Source: CAD feature listing. Evaluate the final solid. Frame: model axes, mm. Face numbers are marked on the shaded views. A direction names the side the tool comes from. Round coordinates to 2 decimals unless told otherwise and drop trailing zeros. Loops run counter-clockwise (first coordinate to the right, second up) from the corner with the lowest first, then second, coordinate; pieces in that order, holes last. Notation, with made-up numbers: M 76,-22 L 103,-22 A22 ccw 103,-8 Z; hole C 41,37 d6. An arc over 180 degrees is marked long. Write each question's results on one line, items separated by ' | '. Start each with the question number.
1. Set-up query: the marked faces 1 and 2. Return all of +Z, -Z, +X, -X, +Y, -Y with unobstructed straight access to the full face (end or side cutting, diameter ignored); none if empty.
2. Section A-A on y = 9. Give the number of separate pieces and of enclosed holes in the cut face, and give its area (3 significant figures).
3. Ray query, line 1 (Z direction, x = -50.5, y = 7.25) (3 decimals); line 2 (Y direction, x = -40.5, z = -7); line 3 (X direction, y = 8.75, z = -10.5) (3 decimals). Return the intervals inside material, ascending.
4. Contact query for flat-ended pins moving along their axis: pin 1 Ø1.6 at (x, y) = (-71, 9.5) entering from -Z (3 decimals); pin 2 Ø3.5 at (x, z) = (-78, -39) entering from +Y; pin 3 Ø3 at (y, z) = (8, -67.5) entering from +X (3 decimals). Output: stop coordinate, or through.
5. Section B-B on z = -12.5. Output: boundary loops of the cut face in (x, y) (3 decimals).
6. Section D-D on z = -36.5. Output: boundary loops of the cut face in (x, y) (3 decimals).
7. Draft query along X for the marked faces 3 and 4. Return one class per face: released by +X, released by -X, zero draft, split by the parting line, or undercut.
Autodesk Inventor part; units mm, degrees
ref_plane "YZ Plane" through (0, 0, 0) normal (1, 0, 0) x (0, 1, 0)
ref_plane "XZ Plane" through (0, 0, 0) normal (0, 1, 0) x (-1, 0, 0)
ref_plane "XY Plane" through (0, 0, 0) normal (0, 0, 1) x (1, 0, 0)
sketch "Boceto1" plane through (0, 0, 0) normal (0, 1, 0) x (-1, 0, 0)
  line L0 (0, 0) -> (80, 0)
  line L1 (80, 0) -> (80, -80)
  line L2 (80, -80) -> (0, -80)
  line L3 (0, -80) -> (0, 0)
  line L4 (10, -70) -> (70, -70)
  line L5 (70, -70) -> (70, -10)
  line L6 (70, -10) -> (10, -10)
  line L7 (10, -10) -> (10, -70)
  line L8 (0, -12.375) -> (80, -12.375)
  line L9 (0, -14.95) -> (80, -14.95)
  line L10 (0, -17.525) -> (80, -17.525)
  line L11 (80, -20.1) -> (0, -20.1)
  line L12 (0, -22.675) -> (80, -22.675)
  line L13 (0, -12.575) -> (80, -12.575)
  line L14 (0, -15.15) -> (80, -15.15)
  line L15 (0, -17.725) -> (80, -17.725)
  line L16 (80, -20.3) -> (0, -20.3)
  line L17 (0, -22.875) -> (80, -22.875)
  line L18 (0, -25.25) -> (80, -25.25)
  line L19 (0, -25.45) -> (80, -25.45)
  line L20 (10, -40) -> (80, -40)
  line L21 (0, -67.625) -> (80, -67.625)
  line L22 (0, -65.05) -> (80, -65.05)
  line L23 (0, -62.475) -> (80, -62.475)
  line L24 (80, -59.9) -> (0, -59.9)
  line L25 (0, -57.325) -> (80, -57.325)
  line L26 (0, -67.425) -> (80, -67.425)
  line L27 (0, -64.85) -> (80, -64.85)
  line L28 (0, -62.275) -> (80, -62.275)
  line L29 (80, -59.7) -> (0, -59.7)
  line L30 (0, -57.125) -> (80, -57.125)
  line L31 (0, -54.75) -> (80, -54.75)
  line L32 (0, -54.55) -> (80, -54.55)
  line L33 (72.625, -7.375) -> (7.375, -7.375)
  line L34 (7.375, -7.375) -> (7.375, -72.625)
  line L35 (7.375, -72.625) -> (72.625, -72.625)
  line L36 (72.625, -72.625) -> (72.625, -7.375)
  line L37 (7.375, 0) -> (0, 0)
  line L38 (7.375, -80) -> (0, -80)
  point P0 (10, -12.375)
  point P1 (70, -12.375)
  point P2 (10, -14.95)
  point P3 (70, -14.95)
  point P4 (10, -17.525)
  point P5 (70, -17.525)
  point P6 (70, -20.1)
  point P7 (10, -20.1)
  point P8 (10, -22.675)
  point P9 (70, -22.675)
  point P10 (10, -12.575)
  point P11 (70, -12.575)
  point P12 (10, -15.15)
  point P13 (70, -15.15)
  point P14 (10, -17.725)
  point P15 (70, -17.725)
  point P16 (70, -20.3)
  point P17 (10, -20.3)
  point P18 (10, -22.875)
  point P19 (70, -22.875)
  point P20 (10, -25.25)
  point P21 (70, -25.25)
  point P22 (10, -25.45)
  point P23 (70, -25.45)
  point P24 (10, -67.625)
  point P25 (70, -67.625)
  point P26 (10, -65.05)
  point P27 (70, -65.05)
  point P28 (10, -62.475)
  point P29 (70, -62.475)
  point P30 (70, -59.9)
  point P31 (10, -59.9)
  point P32 (10, -57.325)
  point P33 (70, -57.325)
  point P34 (10, -67.425)
  point P35 (70, -67.425)
  point P36 (10, -64.85)
  point P37 (70, -64.85)
  point P38 (10, -62.275)
  point P39 (70, -62.275)
  point P40 (70, -59.7)
  point P41 (10, -59.7)
  point P42 (10, -57.125)
  point P43 (70, -57.125)
  point P44 (10, -54.75)
  point P45 (70, -54.75)
  point P46 (10, -54.55)
  point P47 (70, -54.55)
  point P48 (72.625, -12.375)
  point P49 (7.375, -12.375)
  point P50 (72.625, -54.55)
  point P51 (72.625, -25.45)
  point P52 (70, -25.45)
  point P53 (70, -54.55)
  point P54 (7.375, -25.45)
  point P55 (7.375, -54.55)
  point P56 (10, -54.55)
  point P57 (10, -25.45)
  point P58 (10, -67.625)
  point P59 (7.375, -67.625)
  point P60 (72.625, -67.625)
  point P61 (70, -67.625)
  point P62 (7.375, -14.95)
  point P63 (72.625, -14.95)
  point P64 (72.625, -65.05)
  point P65 (70, -65.05)
  point P66 (10, -65.05)
  point P67 (7.375, -65.05)
  point P68 (70, -67.425)
  point P69 (10, -67.425)
  point P70 (10, -12.575)
  point P71 (70, -12.575)
  point P72 (72.625, -64.85)
  point P73 (7.375, -64.85)
  point P74 (7.375, -15.15)
  point P75 (70, -15.15)
  point P76 (7.375, -62.475)
  point P77 (10, -64.85)
  point P78 (10, -62.475)
  point P79 (72.625, -62.475)
  point P80 (70, -62.475)
  point P81 (70, -64.85)
  point P82 (7.375, -17.525)
  point P83 (10, -15.15)
  point P84 (72.625, -17.525)
  point P85 (72.625, -20.1)
  point P86 (7.375, -20.1)
  point P87 (72.625, -59.9)
  point P88 (70, -59.9)
  point P89 (70, -62.275)
  point P90 (10, -62.275)
  point P91 (10, -59.9)
  point P92 (7.375, -59.9)
  point P93 (10, -17.725)
  point P94 (70, -17.725)
  dimension "d0" = 80
  dimension "d1" = 80
  dimension "d2" = 60
  dimension "d3" = 60
  dimension "d4" = 10
  dimension "d5" = 10
  dimension "d6" = 2.375
  dimension "d7" = 0.2
  dimension "d8" = 2.375
  dimension "d9" = 0.2
  dimension "d10" = 0.2
  dimension "d11" = 0.2
  dimension "d12" = 0.2
  dimension "d13" = 2.375
  dimension "d14" = 2.375
  dimension "d15" = 2.375
  dimension "d16" = 2.375
  dimension "d17" = 0.2
  dimension "d35" = 5
extrude "Extrusión1" add sketch "Boceto1" along normal blind 5 contours L0 L1 L8 L36 L33 L34 L3 | L8 L34 L13 L3 | L13 L34 L9 L3 | L34 L33 L36 L8 L5 L6 L7 | L8 L7 L13 L34 | L1 L13 L36 L8 | L13 L7 L9 L34 | L8 L5 L13 L7 | L7 L6 L5 L8 | L1 L9 L36 L13 | L36 L13 L5 L8 | L14 L34 L10 L3 | L13 L5 L9 L7 | L36 L9 L5 L13 | L14 L7 L10 L34 | L1 L10 L36 L14 | L15 L34 L11 L3 | L14 L5 L10 L7 | L36 L10 L5 L14 | L15 L7 L11 L34 | L1 L11 L36 L15 | L16 L34 L12 L3 | L15 L5 L11 L7 | L36 L11 L5 L15 | L16 L7 L12 L34 | L1 L12 L36 L16 | L17 L34 L18 L3 | L16 L5 L12 L7 | L36 L12 L5 L16 | L17 L7 L18 L34 | L1 L18 L36 L17 | L19 L34 L32 L3 | L17 L5 L18 L7 | L36 L18 L5 L17 | L19 L7 L32 L34 | L1 L20 L36 L19 | L31 L34 L30 L3 | L19 L5 L20 L7 | L1 L32 L36 L20 | L36 L20 L5 L19 | L31 L7 L30 L34 | L7 L20 L5 L32 | L36 L32 L5 L20 | L25 L34 L29 L3 | L31 L5 L30 L7 | L1 L30 L36 L31 | L25 L7 L29 L34 | L31 L36 L30 L5 | L24 L34 L28 L3 | L25 L5 L29 L7 | L1 L29 L36 L25 | L24 L7 L28 L34 | L25 L36 L29 L5 | L23 L34 L27 L3 | L24 L5 L28 L7 | L1 L28 L36 L24 | L23 L7 L27 L34 | L24 L36 L28 L5 | L22 L34 L26 L3 | L23 L5 L27 L7 | L1 L27 L36 L23 | L26 L34 L21 L3 | L22 L7 L26 L34 | L23 L36 L27 L5 | L21 L34 L35 L36 L1 L2 L3 | L26 L7 L21 L34 | L22 L5 L26 L7 | L1 L26 L36 L22 | L21 L7 L4 L5 L36 L35 L34 | L26 L5 L21 L7 | L22 L36 L26 L5 | L1 L21 L36 L26 | L21 L5 L4 L7 | L26 L36 L21 L5
sketch "Boceto2" plane through (0, 0, 0) normal (0, -1, 0) x (1, 0, 0)
  line L0 (0, -80) -> (-80, -80)
  line L1 (-80, 0) -> (0, 0)
  line L2 (-80, -80) -> (-80, 0)
  line L3 (-80, 0) -> (0, 0)
  line L4 (-80, -65.05) -> (0, -65.05) construction
  line L5 (0, 0) -> (0, -80)
  line L6 (-80, -80) -> (0, -80)
extrude "Extrusión4" add sketch "Boceto2" along normal blind 3
extrude "Extrusión5" add sketch "Boceto1" along normal blind 10 contours L34 L33 L36 L8 L5 L6 L7 | L8 L7 L13 L34 | L13 L7 L9 L34 | L8 L5 L13 L7 | L7 L6 L5 L8 | L36 L13 L5 L8 | L9 L7 L14 L34 | L13 L5 L9 L7 | L36 L9 L5 L13 | L14 L7 L10 L34 | L9 L5 L14 L7 | L36 L14 L5 L9 | L10 L7 L15 L34 | L14 L5 L10 L7 | L36 L10 L5 L14 | L15 L7 L11 L34 | L10 L5 L15 L7 | L36 L15 L5 L10 | L36 L11 L5 L15 | L19 L7 L32 L34 | L36 L20 L5 L19 | L36 L32 L5 L20 | L24 L7 L28 L34 | L28 L7 L23 L34 | L23 L7 L27 L34 | L28 L5 L23 L7 | L24 L36 L28 L5 | L27 L7 L22 L34 | L23 L5 L27 L7 | L28 L36 L23 L5 | L22 L7 L26 L34 | L27 L5 L22 L7 | L23 L36 L27 L5 | L26 L7 L21 L34 | L22 L5 L26 L7 | L27 L36 L22 L5 | L21 L7 L4 L5 L36 L35 L34 | L26 L5 L21 L7 | L22 L36 L26 L5 | L21 L5 L4 L7 | L26 L36 L21 L5
sketch "Boceto3" plane through (0, 10, 0) normal (0, 1, 0) x (1, 0, 0)
  line L0 (-7.375, 25.45) -> (-7.375, 54.55)
  line L1 (-7.375, 40) -> (-86.5517, 40)
  line L2 (-5, 39.5) -> (-84.1767, 39.5)
  line L3 (-5, 40.5) -> (-84.1767, 40.5)
  line L4 (-10, 54.55) -> (-10, 25.45)
  line L5 (-5, 40.5) -> (-5, 39.5)
  line L6 (-84.1767, 40.5) -> (-84.1767, 39.5)
  point P0 (0, 0)
  point P1 (-10, 40)
  point P2 (-10, 39.5)
  point P3 (-10, 40.5)
  point P4 (-7.375, 39.5)
  point P5 (-7.375, 40.5)
  dimension "d31" = 0.5
  dimension "d32" = 0.5
extrude "Extrusión6" cut sketch "Boceto3" against normal blind 2 contours L2 L4 L1 L0 | L1 L4 L3 L0 | L2 L6 L1 L4 | L1 L6 L3 L4
equation "\"d8\" = d6"
equation "\"d9\" = d7"
equation "\"d10\" = d9"
equation "\"d11\" = d7"
equation "\"d12\" = d7"
equation "\"d13\" = d6"
equation "\"d14\" = d6"
equation "\"d15\" = d6"
equation "\"d16\" = d6"
equation "\"d17\" = d7"
properties part number "Cortador Ancho PDMS4.5"
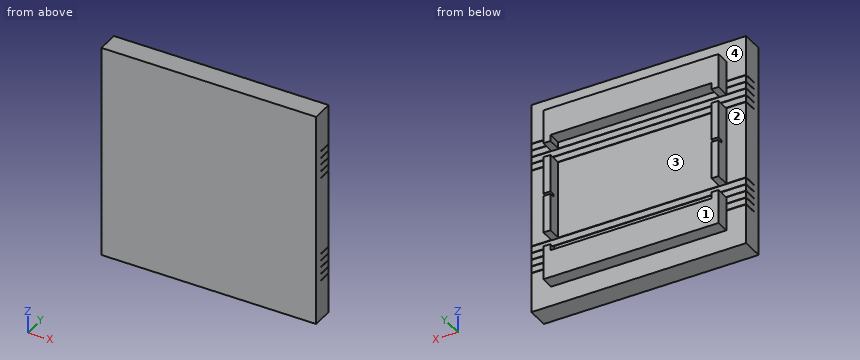
Taken from the geometry:
1) face 1: +Z, -Z, +X, -X, +Y | face 2: +Z, -Z, -X, +Y
2) separate pieces: 6 | enclosed holes: 0 | area: 1,520 mm^2
3) line 1: -72.625 to -62.275, -17.725 to -7.375 | line 2: -3 to 5 | line 3: -72.625 to -7.375
4) pin 1: z = -72.625 | pin 2: y = 5 | pin 3: x = -7.375
5) outline: M -80,-3 L 0,-3 L 0,5 L -7.375,5 L -7.375,10 L -72.625,10 L -72.625,5 L -80,5 Z
6) outline: M -80,-3 L 0,-3 L 0,5 L -7.375,5 L -7.375,10 L -10,10 L -10,5 L -70,5 L -70,10 L -72.625,10 L -72.625,5 L -80,5 Z
7) face 3: undercut | face 4: zero draft
